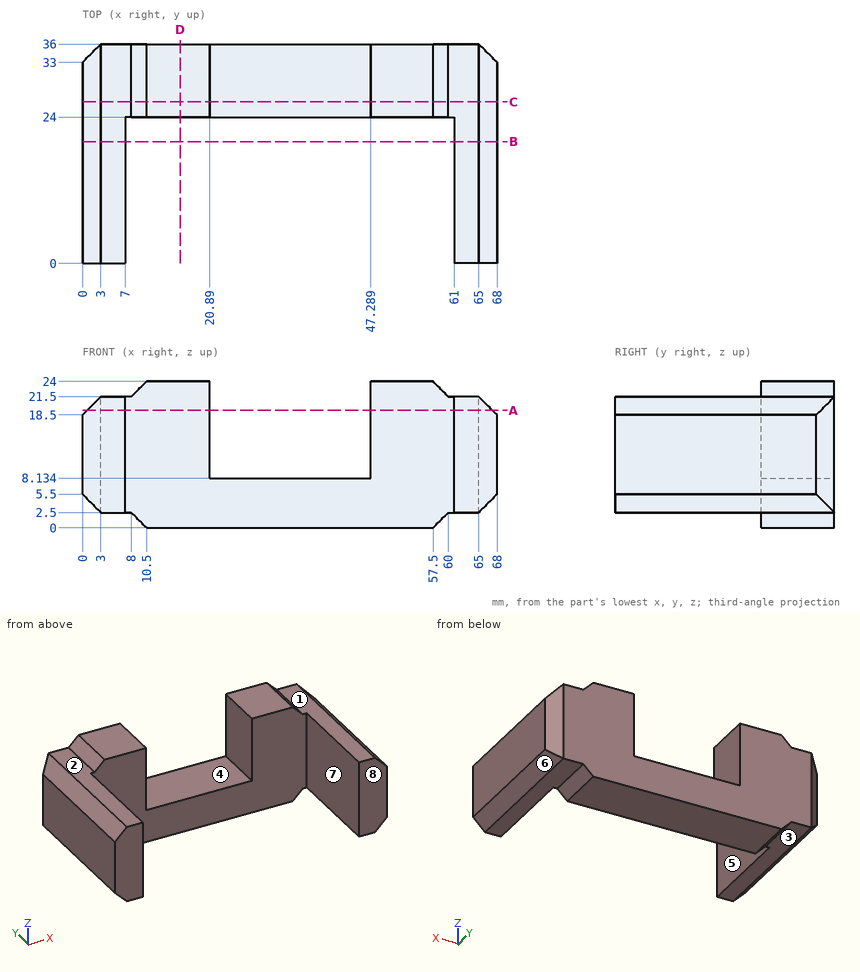
The figure shows three views and two pictorial views of one solid part (mm, origin at its lowest corner). Answer the questions. A direction names the side the tool comes from. Round coordinates to 2 decimals unless told otherwise and drop trailing zeros. Order: outer loops, then holes, each group sorted by start corner. A loop starts at its lowest first (then second) coordinate and runs counter-clockwise, first axis right, second up. Notation, with made-up numbers: (37, 87) -> (94, 87) arc R31 ccw to (94, 121) -> close; hole circle Ø6 at (56.25, 62.25). An arc over 180 degrees is marked (long way). One line per item, written item: value.
Item 1: Given P1, Ø12, axis at x = 49, z = 17, coming from the -Y side; P2, Ø2, axis at y = 13.5, z = 19, coming from the +X side; P3, Ø2.5, axis at x = 62.5, y = 14.5, coming from the -Z side; P4, Ø5.5, axis at x = 6, y = 10, coming from the +Z side, each flat-ended and moving along its own axis, determine where each tip first touches the part or whether it passes through.
Taken from the geometry:
P1: stops at y = 24
P2: stops at x = 68
P3: stops at z = 2.5
P4: stops at z = 21.5
Item 2: Find section D-D, the plane x = 16. Give the vertices of the cut face in (y, z).
Taken from the geometry:
outline: (24, 0) -> (36, 0) -> (36, 24) -> (24, 24) -> close
Item 3: Find section B-B, the plane y = 20. Give the vertices of the cut face in (x, z), then the cut area to 3 significant figures.
Taken from the geometry:
outline: (0, 5.5) -> (3, 2.5) -> (7, 2.5) -> (7, 21.5) -> (3, 21.5) -> (0, 18.5) -> close; (61, 2.5) -> (65, 2.5) -> (68, 5.5) -> (68, 18.5) -> (65, 21.5) -> (61, 21.5) -> close
area: 248 mm2
Item 4: Straight lines are drawn through the part: L1, parallel to X at y = 20.5, z = 16; L2, parallel to X at y = 25, z = 13.75; L3, parallel to Z at x = 5.5, y = 10.5. For each, find the intervals that lie inside material, in ascending order.
Taken from the geometry:
L1: x = 0 to 7, 61 to 68
L2: x = 0 to 20.89, 47.29 to 68
L3: z = 2.5 to 21.5
Item 5: Find section C-C, the plane y = 26.5. Give the vertices of the cut face in (x, z), then the cut area to 3 significant figures.
Taken from the geometry:
outline: (0, 5.5) -> (3, 2.5) -> (8, 2.5) -> (10.5, 0) -> (57.5, 0) -> (60, 2.5) -> (65, 2.5) -> (68, 5.5) -> (68, 18.5) -> (65, 21.5) -> (60, 21.5) -> (57.5, 24) -> (47.29, 24) -> (47.29, 8.13) -> (20.89, 8.13) -> (20.89, 24) -> (10.5, 24) -> (8, 21.5) -> (3, 21.5) -> (0, 18.5) -> close
area: 1,100 mm2
Item 6: For a pull along X with two mould halves and no side action, classify the marked faces 6, 7 and 8 as released by +X, released by -X, zero draft, split by the parting line, or undercut.
Taken from the geometry:
face 6: released by +X
face 7: undercut
face 8: zero draft
Item 7: Find section A-A, the plane z = 19.25. Give the vertices of the cut face in (x, y), then the cut area to 3 significant figures.
Taken from the geometry:
outline: (0.75, 0) -> (7, 0) -> (7, 24) -> (20.89, 24) -> (20.89, 36) -> (3, 36) -> (0.75, 33.75) -> close; (47.29, 24) -> (61, 24) -> (61, 0) -> (67.25, 0) -> (67.25, 33.75) -> (65, 36) -> (47.29, 36) -> close
area: 776 mm2
Item 8: For the marked faces 1, 2, 3, 4 and 5, determine the directions among +Z, -Z, +X, -X, +Y, -Y from which every point of the face is accessible in a straight line to the end or side of a thin tool.
Taken from the geometry:
face 1: +Z, +X, +Y, -Y
face 2: +Z, -X, +Y, -Y
face 3: -Z, -X, +Y, -Y
face 4: +Z, +Y, -Y
face 5: +Z, -Z, -Y
